from build123d import *

# Parameters (mm, degrees)
SKETCH_W        = 62.95
SKETCH_H        = 27.55
PAD_DEPTH       = 2.5
SKETCH001_W     = 60.95
SKETCH001_H     = 25.55
POCKET_DEPTH    = 1
SKETCH002_W     = 8.33494
SKETCH002_H     = 9.82
POCKET001_DEPTH = 5
SKETCH003_W     = 25.55
SKETCH003_H     = 4.198582
POCKET002_DEPTH = 5
SKETCH004_W     = 5.5
SKETCH004_H     = 3.3
SKETCH004_W_2   = 9
SKETCH004_H_2   = 6.6
PAD001_DEPTH    = 1.7
SKETCH005_W     = 9
SKETCH005_H     = 6.6
PAD002_DEPTH    = 1.5
SKETCH006_W     = 11.41477
SKETCH006_H     = 4.37
POCKET003_DEPTH = 1
SKETCH007_R     = 0.9
POCKET004_DEPTH = 5
FILLET_R        = 2
FILLET001_R     = 2
SKETCH008_W     = 30.6
SKETCH008_H     = 1.2
PAD003_DEPTH    = 2.9
FILLET002_R     = 1
SKETCH009_R     = 3.2
SKETCH009_R_2   = 2.5
PAD004_DEPTH    = 1.2
SKETCH010_W     = 1.2
SKETCH010_H     = 9.82
PAD005_DEPTH    = 8.6
PAD006_DEPTH    = 9.8
SKETCH012_W     = 1.01
SKETCH012_H     = 12.1592368492
POCKET005_DEPTH = 5
SKETCH013_W     = 1.919350973
SKETCH013_H     = 0.99
SKETCH013_W_2   = 2.016565973
SKETCH013_H_2   = 1.01
POCKET006_DEPTH = 5
SKETCH014_W     = 3.22658
SKETCH014_H     = 1.4
PAD007_DEPTH    = 7.8
FILLET003_R     = 1
FILLET004_R     = 1
PAD008_DEPTH    = 7.8
SKETCH016_W     = 5.3
SKETCH016_H     = 6.908861
POCKET007_DEPTH = 5
SKETCH017_W     = 7.346396
SKETCH017_H     = 1.27086
POCKET008_DEPTH = 12
FILLET005_R     = 2
FILLET006_R     = 2
SKETCH018_W     = 8.422166
SKETCH018_H     = 10.199767
POCKET009_DEPTH = 31
SKETCH019_R     = 1.5
PAD009_DEPTH    = 7.8
SKETCH020_W     = 10.078106
SKETCH020_H     = 1.351365
POCKET010_DEPTH = 17.076
SKETCH021_R     = 0.9644956182
PAD010_DEPTH    = 7.8


with BuildPart() as part:
    # Sketch → Pad (new body)
    with BuildSketch(Plane.XY):
        Rectangle(SKETCH_W, SKETCH_H)
    extrude(amount=PAD_DEPTH)

    # Sketch001 → Pocket (cut)
    with BuildSketch(Plane.XY.offset(2.5)):
        Rectangle(SKETCH001_W, SKETCH001_H)
    extrude(amount=-POCKET_DEPTH, mode=Mode.SUBTRACT)

    # Sketch002 → Pocket001 (cut)
    with BuildSketch(Plane(origin=(0, 0, 0), x_dir=(1, 0, 0), z_dir=(0, 0, -1))):
        with Locations((-31.64247, 0)):
            Rectangle(SKETCH002_W, SKETCH002_H)
    extrude(amount=-POCKET001_DEPTH, mode=Mode.SUBTRACT)

    # Sketch003 → Pocket002 (cut)
    with BuildSketch(Plane(origin=(30.475, 0, 0), x_dir=(0, -1, 0), z_dir=(-1, 0, 0))):
        with Locations((0, 3.599291)):
            Rectangle(SKETCH003_W, SKETCH003_H)
    extrude(amount=-POCKET002_DEPTH, mode=Mode.SUBTRACT)

    # Sketch004 → Pad001 (new body)
    with BuildSketch(Plane.XY.offset(1.5)):
        with Locations((31.525, 8.3558943219)):
            Rectangle(SKETCH004_W, SKETCH004_H)
        with Locations((31.525, -8.5122186382)):
            Rectangle(SKETCH004_W, SKETCH004_H)
        with Locations((33.275, 0)):
            Rectangle(SKETCH004_W_2, SKETCH004_H_2)
    extrude(amount=PAD001_DEPTH)

    # Sketch005 → Pad002 (new body)
    with BuildSketch(Plane.XY.offset(3.2)):
        with Locations((33.275, 0)):
            Rectangle(SKETCH005_W, SKETCH005_H)
    extrude(amount=PAD002_DEPTH)

    # Sketch006 → Pocket003 (cut)
    with BuildSketch(Plane(origin=(0, 0, 1.5), x_dir=(1, 0, 0), z_dir=(0, 0, -1))):
        with Locations((37.182385, 0.2334771648)):
            Rectangle(SKETCH006_W, SKETCH006_H)
    extrude(amount=-POCKET003_DEPTH, mode=Mode.SUBTRACT)

    # Sketch007 → Pocket004 (cut)
    with BuildSketch(Plane.XY.offset(4.7)):
        with Locations((34.575, 0)):
            Circle(SKETCH007_R)
    extrude(amount=-POCKET004_DEPTH, mode=Mode.SUBTRACT)

    # Fillet
    fillet_edges = [part.edges().sort_by_distance(p)[0] for p in [
        (-31.475, 13.775, 1.25),
        (-31.475, -13.775, 1.25),
    ]]
    fillet(fillet_edges, radius=FILLET_R)

    # Fillet001
    fillet001_edges = [part.edges().sort_by_distance(p)[0] for p in [
        (-30.475, 12.775, 2),
        (-30.475, -12.775, 2),
    ]]
    fillet(fillet001_edges, radius=FILLET001_R)

    # Sketch008 → Pad003 (new body)
    with BuildSketch(Plane.XY.offset(1.5)):
        Rectangle(SKETCH008_W, SKETCH008_H)
    extrude(amount=PAD003_DEPTH)

    # Fillet002
    fillet002_edges = [part.edges().sort_by_distance(p)[0] for p in [
        (15.3, 0, 4.4),
        (-15.3, 0, 4.4),
    ]]
    fillet(fillet002_edges, radius=FILLET002_R)

    # Sketch009 → Pad004 (new body)
    with BuildSketch(Plane.XY.offset(1.5)):
        with Locations((-12.019986846, 7.041554)):
            Circle(SKETCH009_R)
        with Locations((-12.019986846, 7.041554)):
            Circle(SKETCH009_R_2, mode=Mode.SUBTRACT)
        with Locations((11.580013154, 5.839929)):
            Circle(SKETCH009_R)
        with Locations((11.580013154, 5.839929)):
            Circle(SKETCH009_R_2, mode=Mode.SUBTRACT)
        with Locations((12.019994, -7.139266)):
            Circle(SKETCH009_R)
        with Locations((12.019994, -7.139266)):
            Circle(SKETCH009_R_2, mode=Mode.SUBTRACT)
        with Locations((-12.019986846, -7.041554)):
            Circle(SKETCH009_R)
        with Locations((-12.019986846, -7.041554)):
            Circle(SKETCH009_R_2, mode=Mode.SUBTRACT)
    extrude(amount=PAD004_DEPTH)

    # Sketch010 → Pad005 (new body)
    with BuildSketch(Plane.XY.offset(1.5)):
        with Locations((-26.875, 0)):
            Rectangle(SKETCH010_W, SKETCH010_H)
    extrude(amount=PAD005_DEPTH)

    # Sketch011 → Pad006 (new body)
    with BuildSketch(Plane.XZ.offset(4.91)):
        with BuildLine():
            ThreePointArc((-26.275, 10.1), (-27.6188640233, 11.5918517208), (-29.242495409, 10.410575634))
            Line((-29.242495409, 10.410575634), (-31.4457534602, 0))
            Line((-30.2191738146, 0), (-31.4457534602, 0))
            Line((-28.0684990822, 10.1621151248), (-30.2191738146, 0))
            ThreePointArc((-27.475, 10.1), (-27.7437728057, 10.3983703443), (-28.0684990822, 10.1621151248))
            Line((-26.275, 10.1), (-27.475, 10.1))
        make_face()
    extrude(amount=-PAD006_DEPTH)

    # Sketch012 → Pocket005 (cut)
    with BuildSketch(Plane.YZ.offset(-26.275)):
        with Locations((-4.405, 7.5796184246)):
            Rectangle(SKETCH012_W, SKETCH012_H)
        with Locations((4.405, 7.5796184246)):
            Rectangle(SKETCH012_W, SKETCH012_H)
    extrude(amount=-POCKET005_DEPTH, mode=Mode.SUBTRACT)

    # Sketch013 → Pocket006 (cut)
    with BuildSketch(Plane.XY.offset(1.5)):
        with Locations((-30.8613945135, 4.395)):
            Rectangle(SKETCH013_W, SKETCH013_H)
        with Locations((-30.9100020135, -4.405)):
            Rectangle(SKETCH013_W_2, SKETCH013_H_2)
    extrude(amount=-POCKET006_DEPTH, mode=Mode.SUBTRACT)

    # Sketch014 → Pad007 (new body)
    with BuildSketch(Plane.XZ.offset(3.9)):
        with Locations((-31.8324638146, 0.7)):
            Rectangle(SKETCH014_W, SKETCH014_H)
    extrude(amount=-PAD007_DEPTH)

    # Fillet003
    fillet003_edges = [part.edges().sort_by_distance(p)[0] for p in [
        (-33.445754, -3.9, 0.7),
        (-33.445754, 3.9, 0.7),
    ]]
    fillet(fillet003_edges, radius=FILLET003_R)

    # Fillet004
    fillet004_edges = [part.edges().sort_by_distance(p)[0] for p in [
        (-33.445754, 0, 1.4),
    ]]
    fillet(fillet004_edges, radius=FILLET004_R)

    # Sketch015 → Pad008 (new body)
    with BuildSketch(Plane.XZ.offset(3.9)):
        Polygon((-30.7896802325, 3.1), (-32.2896802325, 3.1), (-29.7186114617, 8.1608880977), align=None)
    extrude(amount=-PAD008_DEPTH)

    # Sketch016 → Pocket007 (cut)
    with BuildSketch(Plane(origin=(-30.0976779028, 0, 6.3697679641), x_dir=(0, -1, 0), z_dir=(-0.9783302734, 0, 0.2070504194))):
        with Locations((0, -1.0484965)):
            Rectangle(SKETCH016_W, SKETCH016_H)
    extrude(amount=POCKET007_DEPTH, mode=Mode.SUBTRACT)

    # Sketch017 → Pocket008 (cut)
    with BuildSketch(Plane.YZ.offset(37.775)):
        with Locations((0.176766, 5.13543)):
            Rectangle(SKETCH017_W, SKETCH017_H)
    extrude(amount=-POCKET008_DEPTH, mode=Mode.SUBTRACT)

    # Fillet005
    fillet005_edges = [part.edges().sort_by_distance(p)[0] for p in [
        (31.475, 13.775, 1.25),
    ]]
    fillet(fillet005_edges, radius=FILLET005_R)

    # Fillet006
    fillet006_edges = [part.edges().sort_by_distance(p)[0] for p in [
        (31.475, -13.775, 1.25),
    ]]
    fillet(fillet006_edges, radius=FILLET006_R)

    # Sketch018 → Pocket009 (cut)
    with BuildSketch(Plane.YZ.offset(15.3)):
        with Locations((-6.727006, 7.2998835)):
            Rectangle(SKETCH018_W, SKETCH018_H)
        with Locations((6.727006, 7.2998835)):
            Rectangle(SKETCH018_W, SKETCH018_H)
    extrude(amount=-POCKET009_DEPTH, mode=Mode.SUBTRACT)

    # Sketch019 → Pad009 (new body)
    with BuildSketch(Plane.XZ.offset(3.9)):
        with Locations((-27.775, 10.1)):
            Circle(SKETCH019_R)
    extrude(amount=-PAD009_DEPTH)

    # Sketch020 → Pocket010 (cut, through all)
    with BuildSketch(Plane.XZ.offset(3.3)):
        with Locations((33.352842, 4.6756825)):
            Rectangle(SKETCH020_W, SKETCH020_H)
    extrude(amount=-POCKET010_DEPTH, mode=Mode.SUBTRACT)

    # Sketch021 → Pad010 (new body)
    with BuildSketch(Plane.XZ.offset(3.9)):
        with Locations((-27.9238999046, 8.6772876492)):
            Circle(SKETCH021_R)
    extrude(amount=-PAD010_DEPTH)


solid = part.part
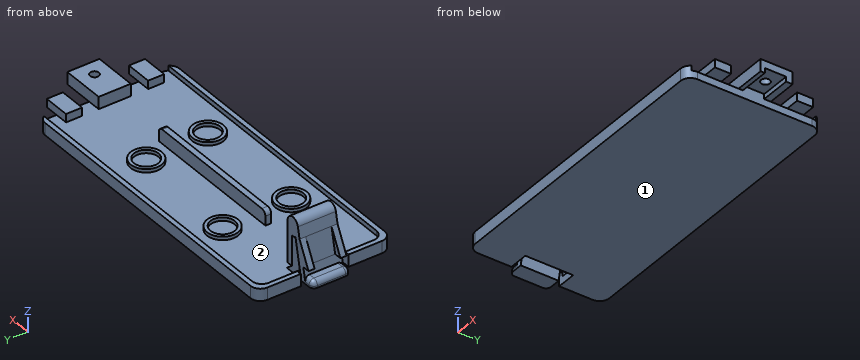
CAD build for the part. Positions are in the model's coordinates, mm. Face numbers are marked on the shaded views. Give positions to 0.01 mm unless a question says otherwise; leave off trailing zeros. Order: outer loops, then holes, each group sorted by start corner. A loop starts at its lowest first (then second) coordinate and runs counter-clockwise, first axis right, second up. Notation, with made-up numbers: (12.25, 9) - (28.25, 9) arc R31 cw to (28.25, 42) - close; hole circle Ø4 at (51.25, 88.5). An arc over 180 degrees is marked (long way). Answer in a Markdown table with one row per item.
1. Saw through at B-B, the plane x = 3. Give the cut face in (y, z) (3 decimals), plus the area to 3 significant figures.
Data:
| item | result |
|---|---|
| outline | (-13.775, 0) - (13.775, 0) - (13.775, 2.5) - (12.775, 2.5) - (12.775, 1.5) - (0.6, 1.5) - (0.6, 4.4) - (-0.6, 4.4) - (-0.6, 1.5) - (-12.775, 1.5) - (-12.775, 2.5) - (-13.775, 2.5) - close |
| area | 46.8 mm² |
2. Flat gauge pins, fed straight in: pin 1 (1.4 mm diameter, centred on x = 31.5, z = 2.5, fed in from -Y); pin 2 (1.5 mm diameter, centred on x = 20.5, z = 3.5, fed in from +Y); pin 3 (6 mm diameter, centred on y = -5.5, z = 7.5, fed in from -X); pin 4 (3 mm diameter, centred on x = -29.5, z = 8, fed in from +Y). Where does each tip first touch, or does it go through?
Data:
| item | result |
|---|---|
| pin 1 | stops at y = -13.27 |
| pin 2 | passes through |
| pin 3 | stops at x = -31.34 |
| pin 4 | stops at y = 3.9 |
3. Probe probe 1 along Y at (x, z) = (32.5, 3); probe 2 along Z at (x, y) = (33, -7.25); probe 3 along Z at (x, y) = (-12.5, 3.25). List the from-to ranges inside material, lowest first. Write a range as [from, to].
Data:
| item | result |
|---|---|
| probe 1 | y = [-10.16, -6.86], [-3.3, 3.3], [6.71, 10.01] |
| probe 2 | z = [1.5, 3.2] |
| probe 3 | z = [0, 1.5] |
4. Saw through at C-C, the plane x = -19. Give the cut face in (y, z) (3 decimals), plus the area to 3 significant figures.
Data:
| item | result |
|---|---|
| outline | (-13.775, 0) - (13.775, 0) - (13.775, 2.5) - (12.775, 2.5) - (12.775, 1.5) - (-12.775, 1.5) - (-12.775, 2.5) - (-13.775, 2.5) - close |
| area | 43.3 mm² |
5. Pull direction X, two halves, no side cores. Call the marked faces 1 and 2: pulls with the +X half, pulls with the -X half, needs draft (parallel to the pull), parting line crosses it, or undercut.
Data:
| item | result |
|---|---|
| face 1 | needs draft |
| face 2 | undercut |
6. Saw through at A-A, the plane z = 7. Give the cut face in (x, y) (3 decimals), plus the area to 3 significant figures.
Data:
| item | result |
|---|---|
| outline | (-30.308, -3.9) - (-28.738, -3.9) - (-28.738, 3.9) - (-30.308, 3.9) - (-30.308, 2.65) - (-29.964, 2.65) - (-29.964, -2.65) - (-30.308, -2.65) - close; (-27.475, -3.9) - (-26.275, -3.9) - (-26.275, 3.9) - (-27.475, 3.9) - close |
| area | 19.8 mm² |
